```python
from build123d import *

# Parameters (mm, degrees)
SKETCH1_W                  = 60
SKETCH1_H                  = 45
BOSS_EXTRUDE1_DEPTH        = 2
F_3_4_3_4_DIAMETER_HOLE1_D = 3.4
SKETCH5_R                  = 2.5
AIR_HOLES_DEPTH            = 76.026661928
CIRPATTERN1_COUNT          = 4
SKETCH6_R                  = 2.5
BOSS_EXTRUDE3_DEPTH        = 2
BOSS_EXTRUDE5_DEPTH        = 3


with BuildPart() as part:
    # Sketch1 → Boss-Extrude1 (new body)
    with BuildSketch(Plane(origin=(0, 0, 0), x_dir=(1, 0, 0), z_dir=(0, 1, 0))):
        with Locations((30, 22.5)):
            Rectangle(SKETCH1_W, SKETCH1_H)
    extrude(amount=BOSS_EXTRUDE1_DEPTH)

    # Ø3.4 (3.4) Diameter Hole1 (through all)
    with Locations(Plane(origin=(0, 2, 0), x_dir=(1, 0, 0), z_dir=(0, 1, 0))):
        with Locations((4, 15), (4, 35), (56, 35), (56, 15)):
            Hole(F_3_4_3_4_DIAMETER_HOLE1_D / 2)

    # Sketch5 → Air holes (cut, through all)
    with BuildSketch(Plane(origin=(0, 2, 0), x_dir=(1, 0, 0), z_dir=(0, 1, 0))):
        with Locations(Location((30, 21, 0), (0, 0, 270))):
            Circle(SKETCH5_R)
        with BuildLine():
            Line((20.507224712, 32.614095631), (23.355142668, 29.766177675))
            ThreePointArc((23.355142668, 29.766177675), (30, 32), (36.644857332, 29.766177675))
            Line((36.644857332, 29.766177675), (39.492775288, 32.614095631))
            ThreePointArc((39.492775288, 32.614095631), (30, 36), (20.507224712, 32.614095631))
        make_face()
        with BuildLine():
            Line((24.785709973, 28.335610371), (27.687975781, 25.433344563))
            ThreePointArc((27.687975781, 25.433344563), (30, 26), (32.312024219, 25.433344563))
            Line((32.312024219, 25.433344563), (35.214290027, 28.335610371))
            ThreePointArc((35.214290027, 28.335610371), (30, 30), (24.785709973, 28.335610371))
        make_face()
        with BuildLine():
            Line((40.913269843, 34.034590187), (43.041644604, 36.162964948))
            ThreePointArc((43.041644604, 36.162964948), (30, 41), (16.958355396, 36.162964948))
            Line((16.958355396, 36.162964948), (19.086730157, 34.034590187))
            ThreePointArc((19.086730157, 34.034590187), (30, 38), (40.913269843, 34.034590187))
        make_face()
    air_holes = extrude(amount=-AIR_HOLES_DEPTH, mode=Mode.SUBTRACT)

    # CirPattern1: Air holes ×4 about axis
    cirpattern1_axis = Axis((30, 0, -21), (0, 1, 0))
    for i in range(1, CIRPATTERN1_COUNT):
        add(air_holes.rotate(cirpattern1_axis, i * 360 / CIRPATTERN1_COUNT), mode=Mode.SUBTRACT)

    # Sketch6 → Boss-Extrude3 (add)
    with BuildSketch(Plane(origin=(0, 2, 0), x_dir=(1, 0, 0), z_dir=(0, 1, 0))):
        with Locations((30, 21)):
            Circle(SKETCH6_R)
    extrude(amount=-BOSS_EXTRUDE3_DEPTH)

    # Sketch10 → Boss-Extrude5 (add)
    with BuildSketch(Plane(origin=(0, 0, -45), x_dir=(-1, 0, 0), z_dir=(0, 0, -1))):
        with BuildLine():
            Line((-60, 2), (-56.468753312, 7.6499947))
            ThreePointArc((-56.468753312, 7.6499947), (-54.652604454, 9.373212406), (-52.228761792, 10))
            Line((-52.228761792, 10), (-7.771238208, 10))
            ThreePointArc((-7.771238208, 10), (-5.347395546, 9.373212406), (-3.531246688, 7.6499947))
            Line((-3.531246688, 7.6499947), (0, 2))
            Line((0, 2), (0, 0))
            Line((0, 0), (-60, 0))
            Line((-60, 0), (-60, 2))
        make_face()
    extrude(amount=-BOSS_EXTRUDE5_DEPTH)


solid = part.part
```
Check sheet for the modelled part. Datum: model origin and axes. Units: mm. A direction names the side the tool comes from. Give positions to 0.01 mm unless a question says otherwise; leave off trailing zeros. Order: outer loops, then holes, each group sorted by start corner. A loop starts at its lowest first (then second) coordinate and runs counter-clockwise, first axis right, second up. Notation, with made-up numbers: M -29.5,-29.5 L 23.5,-29.5 A21 ccw 23.5,-8.5 Z; hole C 24,64 d10. An arc over 180 degrees is marked long. Answer in a Markdown table with one row per item. Add a question column.
Q1. Gauge pin test, flat end, axial feed: pin 1 Ø21 at (x, z) = (39, -20) entering from +Y. Record the tip position at first contact, or that the pin passes through.
Q2. Thickness scan on L1, parallel to Z at x = 4, y = 1.45; L2, parallel to Y at x = 35.5, z = -26; L3, parallel to Z at x = 18, y = 4.25. Record the ranges inside material, lowest first.
Q3. Sectioned sample at C-C, the plane x = 5. Record the boundary of the cut face in (y, z).
Q4. Access from +Z, -Z, +X, -X, +Y, -Y to the whole of each face (thin tool, end or side, straight path). Record for faces 1 (the flat face through (30, 0, -23)), 2 (the flat face through (41.96, 1.01, -35.08)).
Q5. Sectioned sample at B-B, the plane z = -35. Record the boundary of the cut face in (x, y), and give its area (3 significant figures).
Q6. Sectioned sample at D-D, the plane z = -18. Record the boundary of the cut face in (x, y).
Q7. Release check for a two-part mould opening along X. For faces 3 (the cylindrical face through (5.4, 9.4, -43.5)), 4 (the flat face through (30, 6, -42)), 5 (the cylindrical face through (30, 1, -32)) record: released by +X, released by -X, zero draft, split by the parting line, or undercut.
Q8. Sectioned sample at A-A, the plane z = -40. Record the boundary of the cut face in (x, y) (3 decimals), and give its area (3 significant figures).
Verdict:
| question | item | result |
|---|---|---|
| 1 | pin 1 | y = 2 |
| 2 | L1 | -45 to -36.7, -33.3 to -16.7, -13.3 to 0 |
| 2 | L2 | 0 to 2 |
| 2 | L3 | -45 to -42 |
| 3 | outline | M 0,-45 L 9.16,-45 L 9.16,-42 L 2,-42 L 2,-36.37 L 0,-36.37 Z; M 0,-33.63 L 2,-33.63 L 2,-16.37 L 0,-16.37 Z; M 0,-13.63 L 2,-13.63 L 2,0 L 0,0 Z |
| 4 | face 1 | +Z, -Z, +X, -X, -Y |
| 4 | face 2 | +Y, -Y |
| 5 | outline | M 0,0 L 2.3,0 L 2.3,2 L 0,2 Z; M 5.7,0 L 18.12,0 L 18.12,2 L 5.7,2 Z; M 20.36,0 L 24.61,0 L 24.61,2 L 20.36,2 Z; M 35.39,0 L 39.64,0 L 39.64,2 L 35.39,2 Z; M 41.88,0 L 54.3,0 L 54.3,2 L 41.88,2 Z; M 57.7,0 L 60,0 L 60,2 L 57.7,2 Z |
| 5 | area | 75.9 mm² |
| 6 | outline | M 0,0 L 10.23,0 L 10.23,2 L 0,2 Z; M 13.27,0 L 15.3,0 L 15.3,2 L 13.27,2 Z; M 19.42,0 L 21.51,0 L 21.51,2 L 19.42,2 Z; M 24.88,0 L 35.12,0 L 35.12,2 L 24.88,2 Z; M 38.49,0 L 40.58,0 L 40.58,2 L 38.49,2 Z; M 44.7,0 L 46.73,0 L 46.73,2 L 44.7,2 Z; M 49.77,0 L 60,0 L 60,2 L 49.77,2 Z |
| 7 | face 3 | released by -X |
| 7 | face 4 | zero draft |
| 7 | face 5 | undercut |
| 8 | outline | M 0,0 L 23.755,0 L 23.755,2 L 0,2 Z; M 36.245,0 L 60,0 L 60,2 L 36.245,2 Z |
| 8 | area | 95.0 mm² |
